from build123d import *

# Parameters (mm, degrees)
BOSS_EXTRUDE1_DEPTH = 3


with BuildPart() as part:
    # Sketch1 → Boss-Extrude1 (new body)
    with BuildSketch(Plane(origin=(0, 0, 0), x_dir=(1, 0, 0), z_dir=(0, 1, 0))):
        with BuildLine():
            ThreePointArc((-75, 20), (-95, 0), (-75, -20))
            Line((-75, -20), (-75, -5))
            ThreePointArc((-75, -5), (-80, 0), (-75, 5))
            Line((-75, 5), (-75, 20))
        make_face()
        with BuildLine():
            Line((-75, -5), (-75, -20))
            ThreePointArc((-75, -20), (-60.857864376, -14.142135624), (-55, 0))
            ThreePointArc((-55, 0), (-60.857864376, 14.142135624), (-75, 20))
            Line((-75, 20), (-75, 5))
            ThreePointArc((-75, 5), (-71.464466094, 3.535533906), (-70, 0))
            ThreePointArc((-70, 0), (-71.464466094, -3.535533906), (-75, -5))
        make_face()
        with BuildLine():
            ThreePointArc((-55, 0), (-60.857864376, -14.142135624), (-75, -20))
            Line((-75, -20), (75, -20))
            Line((75, -20), (75, 20))
            Line((75, 20), (-75, 20))
            ThreePointArc((-75, 20), (-60.857864376, 14.142135624), (-55, 0))
        make_face()
    extrude(amount=BOSS_EXTRUDE1_DEPTH)


solid = part.part
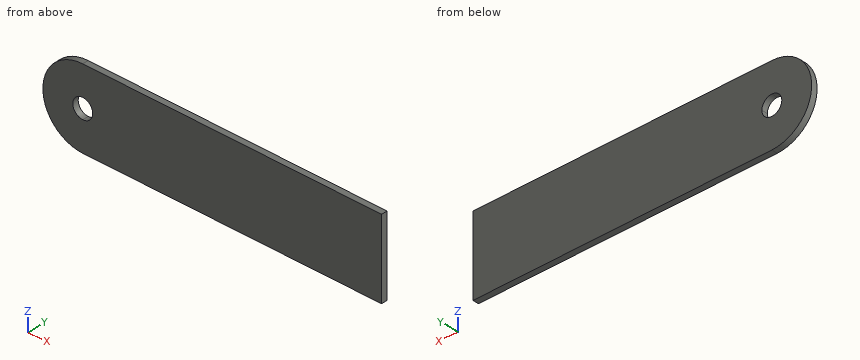
Here's how the part is built. I have some questions about the finished solid (model axes, mm). Give positions to 0.01 mm unless a question says otherwise; leave off trailing zeros. Order: outer loops, then holes, each group sorted by start corner. A loop starts at its lowest first (then second) coordinate and runs counter-clockwise, first axis right, second up. Notation, with made-up numbers: M 56.25,31.5 L 99.25,31.5 A10 cw 99.25,47.5 Z; hole C 33.25,70 d5. An arc over 180 degrees is marked long. Answer as a JSON object with one key per item and string values. Group by question number.
1) I'm going to push a flat-ended pin straight in: pin 1 Ø1 at (y, z) = (1.5, 1.5) entering from -X (3 decimals). Where does the tip first touch, or does it pass through?
2) Suppose I cut it at C-C, the plane z = 13.5. Write out the boundary of the cut face in (x, y), plus the area to 3 significant figures.
3) Suppose I cut it at A-A, the plane y = 1.6. Write out the boundary of the cut face in (x, z), plus the area to 3 significant figures.
4) Please list where these lines run through material, in increasing order: L1, parallel to X at y = 0.25, z = 4; L2, parallel to X at y = 0.8, z = -1; L3, parallel to X at y = 1.5, z = 16. Write a range as [from, to].
5) Suppose I cut it at B-B, the plane z = 3.5. Write out the boundary of the cut face in (x, y), plus the area to 3 significant figures.
Results found:
{
 "1": {"pin 1": "x = -94.975"},
 "2": {"outline": "M -89.76,0 L 75,0 L 75,3 L -89.76,3 Z", "area": "494 mm²"},
 "3": {"outline": "M -75,-20 L 75,-20 L 75,20 L -75,20 A20 ccw Z; hole C -75,0 d10", "area": "6,550 mm²"},
 "4": {"L1": "[-94.6, -78], [-72, 75]", "L2": "[-94.97, -79.9], [-70.1, 75]", "L3": "[-87, 75]"},
 "5": {"outline": "M -94.69,0 L -78.57,0 L -78.57,3 L -94.69,3 Z; M -71.43,0 L 75,0 L 75,3 L -71.43,3 Z", "area": "488 mm²"}
}
